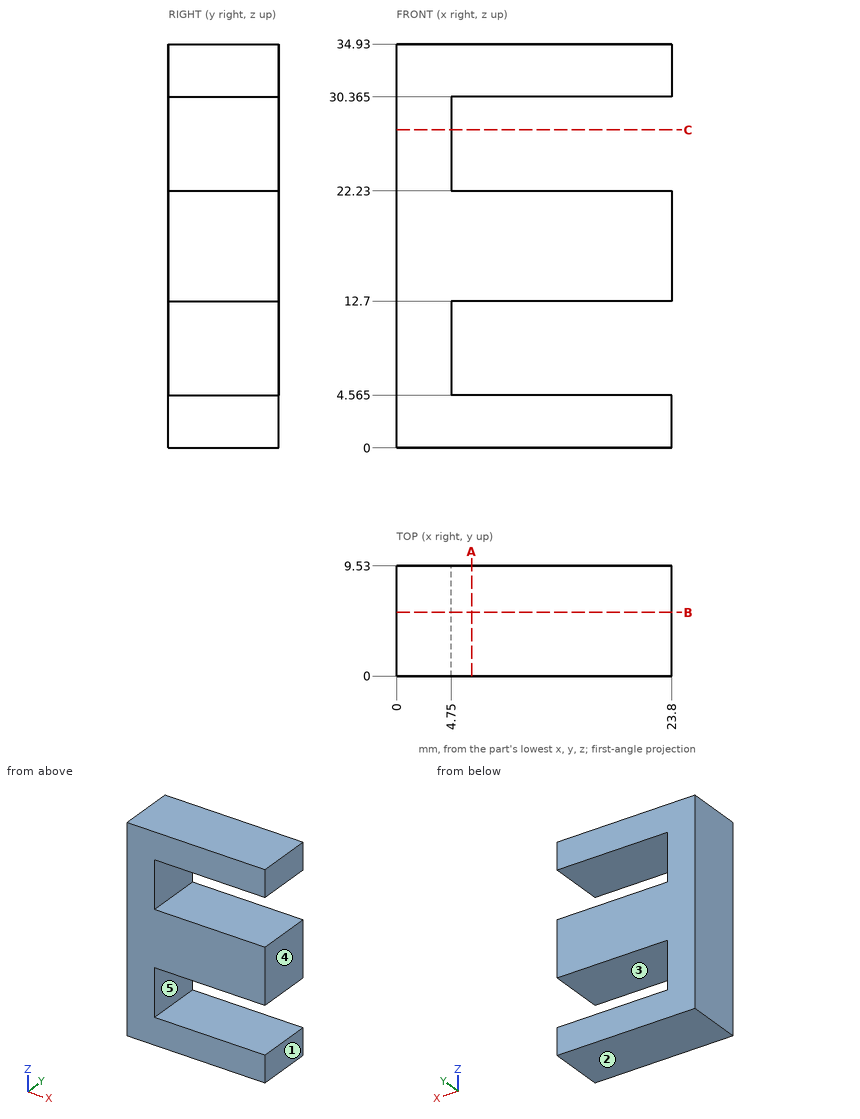
Can you work these out from the drawing? Everything is in mm from the part's minimum corner. A direction names the side the tool comes from. Give positions to 0.01 mm unless a question says otherwise; leave off trailing zeros. Loops run counter-clockwise (first coordinate to the right, second up) from the corner with the lowest first, then second, coordinate; pieces in that order, holes last. Notation, with made-up numbers: (15.5, -1.5) -> (45.5, -1.5) arc R23 cw to (45.5, 23.5) -> close; hole circle Ø6 at (-40, 14). An arc over 180 degrees is marked (long way). Return JSON: item names as keys, results as strings.
Item 1: If we section it at B-B on y = 5.5: List the corners of the cut face in (x, z) for me (3 decimals).
Geometry results:
{"outline": "(0, 0) -> (23.8, 0) -> (23.8, 4.565) -> (4.75, 4.565) -> (4.75, 12.7) -> (23.8, 12.7) -> (23.8, 22.23) -> (4.75, 22.23) -> (4.75, 30.365) -> (23.8, 30.365) -> (23.8, 34.93) -> (0, 34.93) -> close"}
Item 2: Which directions (+Z, -Z, +X, -X, +Y, -Y) give clear straight access to the entire face, cutting with the end or side of a thin tool? Please do the marked faces 4 and 5.
Geometry results:
{"face 4": "+Z, -Z, +X, +Y, -Y", "face 5": "+X, +Y, -Y"}
Item 3: We'd pull the mould along Z, two halves only. Please class the marked faces 1, 2 and 3: +Z half, -Z half, draft (parallel to the pull), parting line (faces both ways), or undercut.
Geometry results:
{"face 1": "draft", "face 2": "-Z half", "face 3": "undercut"}
Item 4: If we section it at C-C on z = 27.5: List the corners of the cut face in (x, y) for me, plus the area to 3 significant figures.
Geometry results:
{"outline": "(0, 0) -> (4.75, 0) -> (4.75, 9.53) -> (0, 9.53) -> close", "area": "45.3 mm²"}
Item 5: I need wall thicknesses on L1, parallel to Z at x = 16.5, y = 5.25 (3 decimals); L2, parallel to X at y = 1, z = 27.5. Which ranges of each line are inside material? Lowest first, please. Write a range as from..to.
Geometry results:
{"L1": "z = 0..4.565, 12.7..22.23, 30.365..34.93", "L2": "x = 0..4.75"}
Item 6: If we section it at A-A on x = 6.5: List the corners of the cut face in (y, z) for me (3 decimals), plus the area to 3 significant figures.
Geometry results:
{"outline": "(0, 0) -> (9.53, 0) -> (9.53, 4.565) -> (0, 4.565) -> close; (0, 12.7) -> (9.53, 12.7) -> (9.53, 22.23) -> (0, 22.23) -> close; (0, 30.365) -> (9.53, 30.365) -> (9.53, 34.93) -> (0, 34.93) -> close", "area": "178 mm²"}
Item 7: I'm going to push a flat-ended pin straight in: pin 1 (2.5 mm diameter, centred on y = 4, z = 8, fed in from +X). Where does the tip first touch, or does it pass through?
Geometry results:
{"pin 1": "stops at x = 4.75"}
